Design review of the part shown in the three views and the two pictorial views. Dimensions are in mm from the part's minimum x, y and z. A direction names the side the tool comes from. Coordinates: 2 decimals unless noted, no trailing zeros. Loops run counter-clockwise (first coordinate to the right, second up) from the corner with the lowest first, then second, coordinate; pieces in that order, holes last. Notation, with made-up numbers: (37, 15) -> (58, 15) arc R12 cw to (58, 20) -> close; hole circle Ø7 at (45, 67.25). An arc over 180 degrees is marked (long way). One line per item, written item: value. Start each with the question number.
1. Add section D-D on z = 6.5. Write out the cut boundary in (x, y), plus the area to 3 significant figures.
2. For probe 1 along Z at (x, y) = (1.75, 5); probe 2 along Z at (x, y) = (1.25, 3); probe 3 along Y at (x, z) = (3, 18.75), list the stretches that pass through material, from the lowest coordinate up.
3. Machinability: for the marked faces 1 and 2, which of the approach directions +Z, -Z, +X, -X, +Y, -Y give a long, thin tool a straight path to every point of the face, cutting with its end or side? Answer none if there is none.
4. Insertion check: pin 1 (1 mm diameter, centred on y = 1, z = 20.5, fed in from -X); pin 2 (1.5 mm diameter, centred on x = 6.5, y = 1, fed in from -Z); pin 3 (4 mm diameter, centred on y = 1, z = 19.5, fed in from +X). Each pin has a flat end and moves straight along its axis. Give the tip position at first contact, or say it passes through.
5. Add section A-A on x = 4. Write out the cut boundary in (y, z).
6. Add section C-C on z = 21.5. Write out the cut boundary in (x, y), plus the area to 3 significant figures.
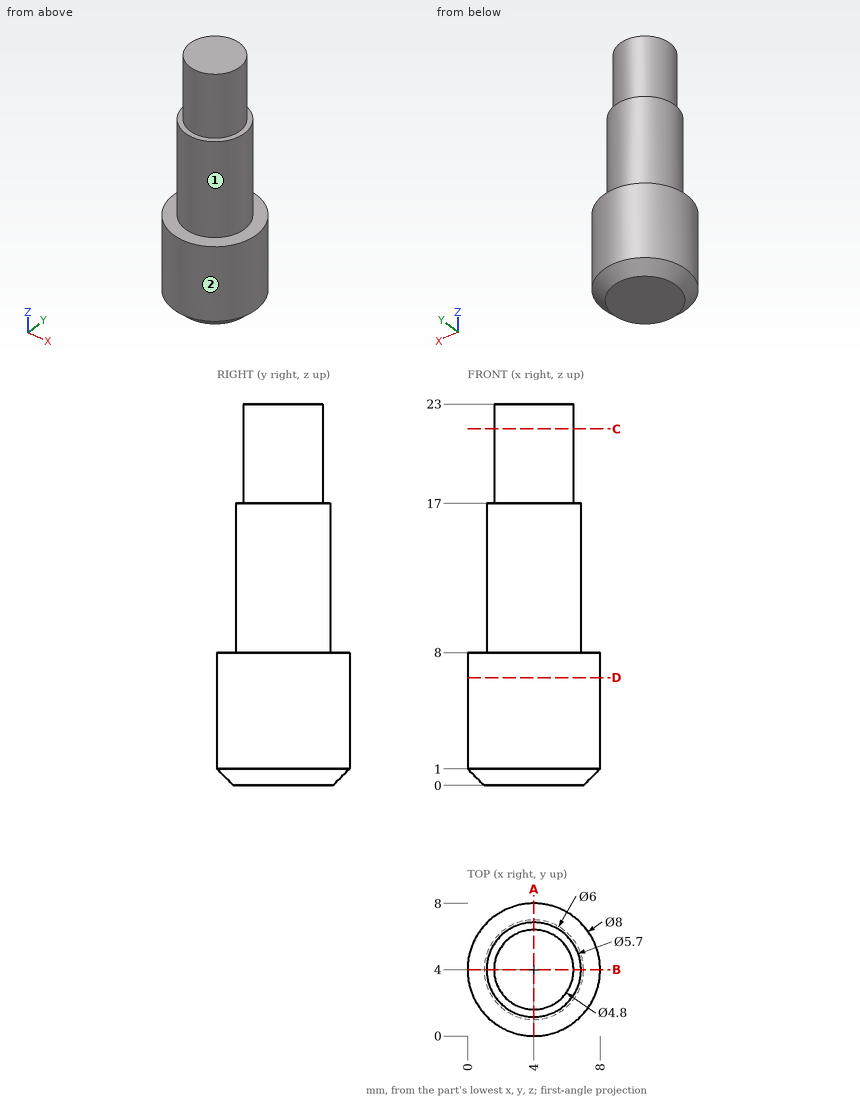
Worked answers:
1. outline: circle Ø8 at (4, 4)
1. area: 50.3 mm²
2. probe 1: z = 0 to 17
2. probe 2: z = 0 to 8
2. probe 3: y = 1.82 to 6.18
3. face 1: +Z
3. face 2: +Z, -Z
4. pin 1: passes through
4. pin 2: stops at z = 0.16
4. pin 3: stops at x = 6.18
5. outline: (0, 1) -> (1, 0) -> (7, 0) -> (8, 1) -> (8, 8) -> (6.85, 8) -> (6.85, 17) -> (6.4, 17) -> (6.4, 23) -> (1.6, 23) -> (1.6, 17) -> (1.15, 17) -> (1.15, 8) -> (0, 8) -> close
6. outline: circle Ø4.8 at (4, 4)
6. area: 18.1 mm²
